For this review, take the finished solid that the model builds, in its own axes (mm). Round coordinates to 2 decimals unless told otherwise and drop trailing zeros. Write each loop counter-clockwise with the first axis right and the second up, starting at its lowest first coordinate (ties: lowest second). Pieces come first, ordered by that corner, then holes. Notation, with made-up numbers: (57.5, 22.25) -> (77.5, 22.25) arc R14 cw to (77.5, 26.25) -> close; hole circle Ø10 at (17.25, 46.25). An arc over 180 degrees is marked (long way). Answer in a Markdown table with one row per item.
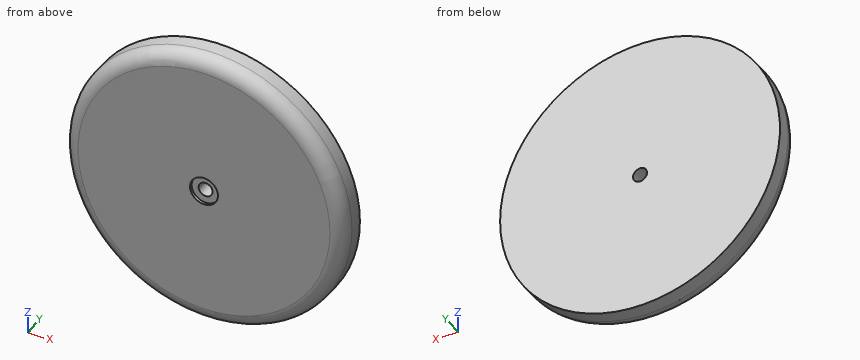
from build123d import *

# Parameters (mm, degrees)
F0_R      = 25
F1_DEPTH  = 5
F2_R      = 2.5
F3_R      = 2.5
F3_R_2    = 1.25
F4_DEPTH  = 0.5
F4_FACE_R = 1.25
F5_DEPTH  = 32.62


with BuildPart() as f1:
    # F0 (on Front) → F1 (new body)
    with BuildSketch(Plane.XZ):
        Circle(F0_R)
    extrude(amount=F1_DEPTH)

    # F2
    f2_edges = [f1.edges().sort_by_distance(p)[0] for p in [
        (-25, -5, 0),
    ]]
    fillet(f2_edges, radius=F2_R)

    # F3 (on face) → F4 (cut)
    with BuildSketch(Plane.XZ.offset(5)):
        Circle(F3_R)
        Circle(F3_R_2, mode=Mode.SUBTRACT)
    extrude(amount=-F4_DEPTH, mode=Mode.SUBTRACT)

    # F4_face (on face) → F5 (cut)
    with BuildSketch(Plane.XZ.offset(5)):
        Circle(F4_FACE_R)
    extrude(amount=-F5_DEPTH, mode=Mode.SUBTRACT)


solid = f1.part
1) For line 1 (Z direction, x = 0, y = -2.1); line 2 (Z direction, x = 0, y = -4.65); line 3 (Z direction, x = 14, y = -2.5), list the stretches that pass through material, from the lowest coordinate up. Write a range as [from, to].
Solved:
| item | result |
|---|---|
| line 1 | [-25, -1.25], [1.25, 25] |
| line 2 | [-23.78, -2.5], [2.5, 23.78] |
| line 3 | [-20.71, 20.71] |
2) Consider section C-C on y = -3.7. State the section outline as (x, z) points, then the cut area to 3 significant figures.
Solved:
| item | result |
|---|---|
| outline | circle Ø49.39 at (0, 0); hole circle Ø2.5 at (0, 0) |
| area | 1,910 mm² |
3) Clearance check with flat-ended pins moving along their axes: pin 1 Ø2 at (y, z) = (-3, 12.5) entering from -X; pin 2 Ø3 at (x, y) = (6.5, -1.5) entering from +Z; pin 3 Ø4 at (x, z) = (0, 0) entering from -Y. State where each tip first meets the part, or that it passes through.
Solved:
| item | result |
|---|---|
| pin 1 | x = -22.17 |
| pin 2 | z = 24.49 |
| pin 3 | y = -4.5 |
4) Consider section B-B on x = 0. State the section outline as (y, z) points, then the cut area to 3 significant figures.
Solved:
| item | result |
|---|---|
| outline | (-5, -22.5) arc R2.5 ccw to (-2.5, -25) -> (0, -25) -> (0, -1.25) -> (-4.5, -1.25) -> (-4.5, -2.5) -> (-5, -2.5) -> close; (-5, 2.5) -> (-4.5, 2.5) -> (-4.5, 1.25) -> (0, 1.25) -> (0, 25) -> (-2.5, 25) arc R2.5 ccw to (-5, 22.5) -> close |
| area | 234 mm² |
5) Consider section A-A on z = 0. State the section outline as (x, y) points.
Solved:
| item | result |
|---|---|
| outline | (-25, -2.5) arc R2.5 ccw to (-22.5, -5) -> (-2.5, -5) -> (-2.5, -4.5) -> (-1.25, -4.5) -> (-1.25, 0) -> (-25, 0) -> close; (1.25, -4.5) -> (2.5, -4.5) -> (2.5, -5) -> (22.5, -5) arc R2.5 ccw to (25, -2.5) -> (25, 0) -> (1.25, 0) -> close |
